Print and shaded views of the part. All mm, measured from the part's lowest x, y and z. A direction names the side the tool comes from. Round coordinates to 2 decimals unless told otherwise and drop trailing zeros. Order: outer loops, then holes, each group sorted by start corner. A loop starts at its lowest first (then second) coordinate and runs counter-clockwise, first axis right, second up. Notation, with made-up numbers: M 16.5,19 L 45.5,19 A12 ccw 45.5,29 Z; hole C 12.25,88.5 d1. An arc over 180 degrees is marked long. Use CSV: the item, a comma, the result in double quotes.
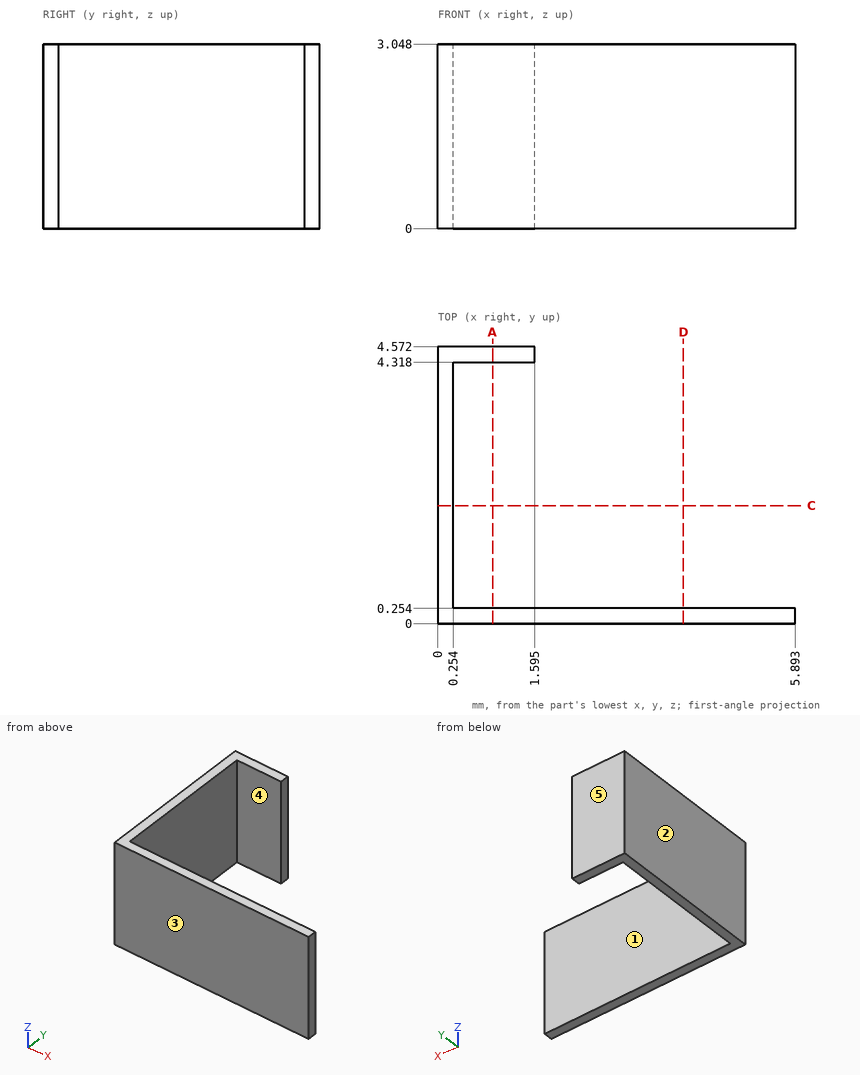
(1) Two-plate mould, pull along Y, no slides. Class the marked faces 3, 4 and 5: released by +Y, released by -Y, zero draft, split by the parting line, or undercut.
Answer block:
face 3,"released by -Y"
face 4,"undercut"
face 5,"released by +Y"
(2) Wall check: line 1 (Y direction, x = 0.55, z = 2.45); line 2 (X direction, y = 3.75, z = 0.35). Give the ranges that are in metal, low to high. Write a range as from..to.
Answer block:
line 1,"y = 0..0.25, 4.32..4.57"
line 2,"x = 0..0.25"
(3) Drop a flat-ended pin along its axis: pin 1 (1.5 mm diameter, centred on y = 3.5, z = 1.5, fed in from +X). Give the stop position or say it passes through.
Answer block:
pin 1,"stops at x = 0.25"
(4) Cut at A-A, the plane x = 0.9. Give the cut face in (y, z).
Answer block:
outline,"M 0,0 L 0.25,0 L 0.25,3.05 L 0,3.05 Z; M 4.32,0 L 4.57,0 L 4.57,3.05 L 4.32,3.05 Z"
(5) Cut at C-C, the plane y = 1.95. Give the cut face in (x, z).
Answer block:
outline,"M 0,0 L 0.25,0 L 0.25,3.05 L 0,3.05 Z"
(6) Tool access for the marked faces 1 and 2: list every direction of +Z, -Z, +X, -X, +Y, -Y with a clear straight run to the whole face (end or side of a thin tool).
Answer block:
face 1,"+Z, -Z, +X"
face 2,"+Z, -Z, -X, +Y, -Y"
